Source: CAD feature listing. Evaluate the final solid. Frame: model axes, mm. A direction names the side the tool comes from. Give positions to 0.01 mm unless a question says otherwise; leave off trailing zeros. Order: outer loops, then holes, each group sorted by start corner. A loop starts at its lowest first (then second) coordinate and runs counter-clockwise, first axis right, second up. Notation, with made-up numbers: (45, 15) - (58, 15) arc R22 ccw to (58, 45) - close; hole circle Ø9 at (-3.75, 62.25). An arc over 180 degrees is marked (long way). Write each question's results on one line, items separated by ' | '. Start each with the question number.
Item 1: Mould query, pull axis X, two halves, no side actions, for faces 4 (the flat face through (4, -7, 10)), 5 (the cylindrical face through (-59.26, -6.54, 3.94)), 6 (the cylindrical face through (-45.704, 4.261, 9.399)), 7 (the cylindrical face through (68.993, -7.157, 3.944)). Classes: released by +X, released by -X, zero draft, split by the parting line, or undercut.
Item 2: Line query: line 1 along Y through (x, z) = (-41, 4.5); line 2 along X through (y, z) = (5.5, 4.25); line 3 along X through (y, z) = (-7, 8). Output: solid intervals per line, ascending.
Item 3: Section A-A on z = 2.5. Output: boundary loops of the cut face in (x, y), and give its area (3 significant figures).
Item 4: Section B-B on x = 23.5. Output: boundary loops of the cut face in (y, z), and give its area (3 significant figures).
Item 5: Set-up query: faces 1 (the flat face through (4, 3.153, 4)), 2 (the cylindrical face through (-45.704, -17.869, 9.399)), 3 (the cylindrical face through (5.59, 2.58, 9.4)). Return all of +Z, -Z, +X, -X, +Y, -Y with unobstructed straight access to the full face (end or side cutting, diameter ignored); none if empty.
Item 6: Contact query for flat-ended pins moving along their axis: pin 1 Ø5 at (x, z) = (-18, 2.5) entering from +Y; pin 2 Ø3.5 at (y, z) = (-19, 4) entering from +X; pin 3 Ø4 at (x, z) = (13, 5) entering from -Y. Output: stop coordinate, or through.
```python
from build123d import *

# Parameters (mm, degrees)
F0_W     = 100
F0_H     = 20
F1_DEPTH = 10
F2_R     = 2


with BuildPart() as f1:
    # F0 (on Top) → F1 (new body)
    with BuildSketch(Plane.XY):
        with BuildLine():
            Line((-45.133696, -16.846582), (-45.133696, 3.153418))
            Line((-45.133696, 3.153418), (-45.133696, 7.283418))
            ThreePointArc((-45.133696, 7.283418), (-59.263696, -6.846582), (-45.133696, -20.976582))
            Line((-45.133696, -20.976582), (-45.133696, -16.846582))
        make_face()
        with Locations((4.866304, -6.846582)):
            Rectangle(F0_W, F0_H)
        with BuildLine():
            Line((54.866304, 7.283418), (54.866304, 3.153418))
            Line((54.866304, 3.153418), (54.866304, -16.846582))
            Line((54.866304, -16.846582), (54.866304, -20.976582))
            ThreePointArc((54.866304, -20.976582), (68.996304, -6.846582), (54.866304, 7.283418))
        make_face()
    extrude(amount=F1_DEPTH)

    # F2
    f2_edges = [f1.edges().sort_by_distance(p)[0] for p in [
        (-45.133696, 5.218418, 10),
        (-45.133696, -18.911582, 10),
        (-59.263696, -6.846582, 10),
        (4.866304, 3.153418, 10),
        (4.866304, -16.846582, 10),
        (68.996304, -6.846582, 10),
        (54.866304, 5.218418, 10),
        (54.866304, -18.911582, 10),
    ]]
    fillet(f2_edges, radius=F2_R)


solid = f1.part
```
Evaluation:
1) face 4: zero draft | face 5: released by -X | face 6: undercut | face 7: released by +X
2) line 1: y = -16.85 to 3.15 | line 2: x = -52.01 to -45.13, 54.87 to 61.74 | line 3: x = -59.26 to 69
3) outline: (-45.13, -20.98) - (-45.13, -16.85) - (54.87, -16.85) - (54.87, -20.98) arc R14.13 ccw to (54.87, 7.28) - (54.87, 3.15) - (-45.13, 3.15) - (-45.13, 7.28) arc R14.13 ccw to start | area: 2,630 mm^2
4) outline: (-16.85, 0) - (3.15, 0) - (3.15, 8) arc R2 ccw to (1.15, 10) - (-14.85, 10) arc R2 ccw to (-16.85, 8) - close | area: 198 mm^2
5) face 1: +Z, -Z, +Y | face 2: +Z, -Y | face 3: +Z, +Y
6) pin 1: stops at y = 3.15 | pin 2: stops at x = 64.43 | pin 3: stops at y = -16.85
